The model under review builds one solid part; all positions refer to its coordinate system, in mm. A direction names the side the tool comes from. Give positions to 0.01 mm unless a question says otherwise; leave off trailing zeros. Write each loop counter-clockwise with the first axis right and the second up, starting at its lowest first coordinate (ties: lowest second). Pieces come first, ordered by that corner, then holes. Notation, with made-up numbers: (-15.75, 56) -> (19.25, 56) arc R24 ccw to (19.25, 68) -> close; hole circle Ø7 at (7.25, -2.75). An arc over 180 degrees is marked (long way). Use CSV: the item, a comma, the result in double quotes.
```python
from build123d import *

# Parameters (mm, degrees)
BOSS_EXTRUDE1_DEPTH                               = 38.1
BOSS_EXTRUDE1_2_DEPTH                             = 38.1
SKETCH1_4_W                                       = 142.24
SKETCH1_4_H                                       = 53.34
BOSS_EXTRUDE2_DEPTH                               = 6.35
SKETCH1_5_W                                       = 142.24
SKETCH1_5_H                                       = 6.35
BOSS_EXTRUDE3_DEPTH                               = 17.78
FILLET1_R                                         = 3.81
CSK_FOR_8_FLAT_HEAD_MACHINE_SCREW_100_D           = 4.4958
CSK_FOR_8_FLAT_HEAD_MACHINE_SCREW_100_CSINK_D     = 8.4328
CSK_FOR_8_FLAT_HEAD_MACHINE_SCREW_100_CSINK_ANGLE = 100


with BuildPart() as part:
    # Sketch1 → Boss-Extrude1 (new body)
    with BuildSketch(Plane(origin=(0, 0, 0), x_dir=(1, 0, 0), z_dir=(0, 1, 0))):
        Polygon((72.784549316, 28.417821782), (72.784549316, 22.067821782), (72.784549316, -31.272178218), (72.784549316, -37.622178218), (79.134549316, -37.622178218), (79.134549316, 28.417821782), align=None)
    extrude(amount=BOSS_EXTRUDE1_DEPTH)



with BuildPart() as body_2:
    # Sketch1 → Boss-Extrude1 2 (new body)
    with BuildSketch(Plane(origin=(0, 0, 0), x_dir=(1, 0, 0), z_dir=(0, 1, 0))):
        Polygon((-69.455450684, -31.272178218), (-69.455450684, 22.067821782), (-69.455450684, 28.417821782), (-75.805450684, 28.417821782), (-75.805450684, -37.622178218), (-69.455450684, -37.622178218), align=None)
    extrude(amount=BOSS_EXTRUDE1_2_DEPTH)


with BuildPart() as part_1:
    add(part.part)

    add(body_2.part)  # Boss-Extrude2 merges body 2
    # Sketch1<4> → Boss-Extrude2 (add)
    with BuildSketch(Plane(origin=(0, 0, 0), x_dir=(1, 0, 0), z_dir=(0, 1, 0))):
        with Locations((1.664549316, -4.602178218)):
            Rectangle(SKETCH1_4_W, SKETCH1_4_H)
    extrude(amount=BOSS_EXTRUDE2_DEPTH)

    # Sketch1<5> → Boss-Extrude3 (add)
    with BuildSketch(Plane(origin=(0, 0, 0), x_dir=(1, 0, 0), z_dir=(0, 1, 0))):
        with Locations((1.664549316, 25.242821782)):
            Rectangle(SKETCH1_5_W, SKETCH1_5_H)
        with Locations((1.664549316, -34.447178218)):
            Rectangle(SKETCH1_5_W, SKETCH1_5_H)
    extrude(amount=BOSS_EXTRUDE3_DEPTH)

    # Fillet1
    fillet1_edges = [part_1.edges().sort_by_distance(p)[0] for p in [
        (75.959549316, 38.1, 37.622178218),
        (75.959549316, 38.1, -28.417821782),
        (-72.630450684, 38.1, -28.417821782),
        (-72.630450684, 38.1, 37.622178218),
        (-69.455450684, 17.78, -25.242821782),
        (72.784549316, 17.78, -25.242821782),
        (72.784549316, 17.78, 34.447178218),
        (-69.455450684, 17.78, 34.447178218),
    ]]
    fillet(fillet1_edges, radius=FILLET1_R)

    # CSK for #8 Flat Head Machine Screw (100)2 (through all)
    with Locations(Plane(origin=(0, 6.35, 0), x_dir=(1, 0, 0), z_dir=(0, 1, 0))):
        with Locations((-45.960450684, -16.032178218), (-45.960450684, 6.827821782), (49.289549316, 6.827821782), (49.289549316, -16.032178218)):
            CounterSinkHole(CSK_FOR_8_FLAT_HEAD_MACHINE_SCREW_100_D / 2, CSK_FOR_8_FLAT_HEAD_MACHINE_SCREW_100_CSINK_D / 2, counter_sink_angle=CSK_FOR_8_FLAT_HEAD_MACHINE_SCREW_100_CSINK_ANGLE)


solid = part_1.part
```
Q1. Insertion check: pin 1 (1 mm diameter, centred on x = -2, z = -14.5, fed in from -Y); pin 2 (6 mm diameter, centred on x = 49.29, z = 16.03, fed in from +Y); pin 3 (3 mm diameter, centred on x = 1, z = -26.5, fed in from +Y). Each pin has a flat end and moves straight along its axis. Give the tip position at first contact, or say it passes through.
Derived:
pin 1,"stops at y = 0"
pin 2,"stops at y = 5.33"
pin 3,"stops at y = 17.78"
Q2. To check wall thickness, follow probe 1 along Z at (x, y) = (17.5, 12); probe 2 along X at (y, z) = (23.5, -1); probe 3 along Y at (x, z) = (-12, 16). State the ranges of each line that lie inside material, in increasing order.
Derived:
probe 1,"z = -28.42 to -22.07, 31.27 to 37.62"
probe 2,"x = -75.81 to -69.46, 72.78 to 79.13"
probe 3,"y = 0 to 6.35"
Q3. Machinability: for faces 1 (the flat face through (72.785, 22, 4)), 2 (the flat face through (1, 17.78, -25)), 3 (the cylindrical face through (47.2, 2.3, -6)), which of the approach directions +Z, -Z, +X, -X, +Y, -Y give a long, thin tool a straight path to every point of the face, cutting with its end or side? Answer none if there is none.
Derived:
face 1,"+Y"
face 2,"+Z, -Z, +Y"
face 3,"+Y, -Y"
Q4. Consider section B-B (y = 11). Write out the cut boundary in (x, z), then the cut area to 3 significant figures.
Derived:
outline,"(-75.81, -28.42) -> (79.13, -28.42) -> (79.13, 37.62) -> (-75.81, 37.62) -> close; hole (-69.46, -22.07) -> (72.78, -22.07) -> (72.78, 31.27) -> (-69.46, 31.27) -> close"
area,"2,650 mm2"
Q5. Consider section C-C (x = 12.5). Write out the cut boundary in (y, z), then the cut area to 3 significant figures.
Derived:
outline,"(0, -28.42) -> (17.78, -28.42) -> (17.78, -22.07) -> (6.35, -22.07) -> (6.35, 31.27) -> (17.78, 31.27) -> (17.78, 37.62) -> (0, 37.62) -> close"
area,"565 mm2"
Q6. Consider section A-A (y = 32). Write out the cut boundary in (x, z), then the cut area to 3 significant figures.
Derived:
outline,"(-75.81, -28.42) -> (-69.46, -28.42) -> (-69.46, 37.62) -> (-75.81, 37.62) -> close; (72.78, -28.42) -> (79.13, -28.42) -> (79.13, 37.62) -> (72.78, 37.62) -> close"
area,"839 mm2"
Q7. The part is to be moulded in two halves that separate along X. For faces 4 (the flat face through (1, 6.35, 4)), 5 (the cylindrical face through (71.64, 18.87, 34.4)), 6 (the flat face through (-73, 38.1, 4)), say which applies: pulls with the +X half, pulls with the -X half, needs draft (parallel to the pull), parting line crosses it, or undercut.
Derived:
face 4,"undercut"
face 5,"undercut"
face 6,"needs draft"
Q8. Consider section D-D (z = -20.5). Write out the cut boundary in (x, y), then the cut area to 3 significant figures.
Derived:
outline,"(-75.81, 0) -> (79.13, 0) -> (79.13, 38.1) -> (72.78, 38.1) -> (72.78, 6.35) -> (-69.46, 6.35) -> (-69.46, 38.1) -> (-75.81, 38.1) -> close"
area,"1,390 mm2"
